```python
from build123d import *

# Parameters (mm, degrees)
BOSS_EXTRUDE1_DEPTH = 3.302
SKETCH3_R           = 5.08
CUT_EXTRUDE1_DEPTH  = 1.651
BOSS_EXTRUDE2_DEPTH = 4.445
SKETCH5_R           = 1.4605
BOSS_EXTRUDE3_DEPTH = 12.7


with BuildPart() as part:
    # Sketch1 → Boss-Extrude1 (new body)
    with BuildSketch(Plane(origin=(0, 0, 0), x_dir=(1, 0, 0), z_dir=(0, 1, 0))):
        with BuildLine():
            ThreePointArc((42.545, -8.433720508), (42.325290161, -7.400350502), (41.704170418, -6.545753376))
            Line((41.704170418, -6.545753376), (11.519480965, 20.620467131))
            ThreePointArc((11.519480965, 20.620467131), (10.730300515, 21.103895846), (9.820310547, 21.2725))
            Line((9.820310547, 21.2725), (-9.820310547, 21.2725))
            ThreePointArc((-9.820310547, 21.2725), (-10.730300515, 21.103895846), (-11.519480965, 20.620467131))
            Line((-11.519480965, 20.620467131), (-41.704170418, -6.545753376))
            ThreePointArc((-41.704170418, -6.545753376), (-42.325290161, -7.400350502), (-42.545, -8.433720508))
            Line((-42.545, -8.433720508), (-42.545, -16.8275))
            ThreePointArc((-42.545, -16.8275), (-41.243089642, -19.970589642), (-38.1, -21.2725))
            Line((-38.1, -21.2725), (-29.845, -21.2725))
            ThreePointArc((-29.845, -21.2725), (-26.701910358, -19.970589642), (-25.4, -16.8275))
            Line((-25.4, -16.8275), (-25.4, -16.3195))
            ThreePointArc((-25.4, -16.3195), (-23.912102448, -12.727397552), (-20.32, -11.2395))
            Line((-20.32, -11.2395), (-8.505751918, -11.2395))
            ThreePointArc((-8.505751918, -11.2395), (-7.87713399, -11.499882072), (-7.616751918, -12.1285))
            Line((-7.616751918, -12.1285), (-7.616751918, -15.9385))
            ThreePointArc((-7.616751918, -15.9385), (-7.505159602, -16.207907684), (-7.235751918, -16.3195))
            Line((-7.235751918, -16.3195), (6.099248082, -16.3195))
            ThreePointArc((6.099248082, -16.3195), (6.368655765, -16.207907684), (6.480248082, -15.9385))
            Line((6.480248082, -15.9385), (6.480248082, -12.1285))
            ThreePointArc((6.480248082, -12.1285), (6.740630153, -11.499882072), (7.369248082, -11.2395))
            Line((7.369248082, -11.2395), (20.32, -11.2395))
            ThreePointArc((20.32, -11.2395), (23.912102448, -12.727397552), (25.4, -16.3195))
            Line((25.4, -16.3195), (25.4, -16.8275))
            ThreePointArc((25.4, -16.8275), (26.701910358, -19.970589642), (29.845, -21.2725))
            Line((29.845, -21.2725), (38.1, -21.2725))
            ThreePointArc((38.1, -21.2725), (41.243089642, -19.970589642), (42.545, -16.8275))
            Line((42.545, -16.8275), (42.545, -8.433720508))
        make_face()
        with BuildLine():
            ThreePointArc((-38.735, -9.8425), (-38.288630735, -8.764869265), (-37.211, -8.3185))
            Line((-37.211, -8.3185), (-30.607, -8.3185))
            ThreePointArc((-30.607, -8.3185), (-29.529369265, -8.764869265), (-29.083, -9.8425))
            Line((-29.083, -9.8425), (-29.083, -16.1925))
            ThreePointArc((-29.083, -16.1925), (-29.529369265, -17.270130735), (-30.607, -17.7165))
            Line((-30.607, -17.7165), (-37.211, -17.7165))
            ThreePointArc((-37.211, -17.7165), (-38.288630735, -17.270130735), (-38.735, -16.1925))
            Line((-38.735, -16.1925), (-38.735, -9.8425))
        make_face(mode=Mode.SUBTRACT)
        with BuildLine():
            Line((30.734, -8.3185), (37.338, -8.3185))
            ThreePointArc((37.338, -8.3185), (38.415630735, -8.764869265), (38.862, -9.8425))
            Line((38.862, -9.8425), (38.862, -16.1925))
            ThreePointArc((38.862, -16.1925), (38.415630735, -17.270130735), (37.338, -17.7165))
            Line((37.338, -17.7165), (30.734, -17.7165))
            ThreePointArc((30.734, -17.7165), (29.656369265, -17.270130735), (29.21, -16.1925))
            Line((29.21, -16.1925), (29.21, -9.8425))
            ThreePointArc((29.21, -9.8425), (29.656369265, -8.764869265), (30.734, -8.3185))
        make_face(mode=Mode.SUBTRACT)
    extrude(amount=BOSS_EXTRUDE1_DEPTH)

    # Sketch3 → Cut-Extrude1 (cut)
    with BuildSketch(Plane(origin=(0, 3.302, 0), x_dir=(1, 0, 0), z_dir=(0, 1, 0))):
        with Locations(Location((-9.9695, 8.8265, 0), (0, 0, 270))):
            Circle(SKETCH3_R)
        with Locations(Location((9.9695, 8.8265, 0), (0, 0, 270))):
            Circle(SKETCH3_R)
    extrude(amount=-CUT_EXTRUDE1_DEPTH, mode=Mode.SUBTRACT)

    # Sketch4 → Boss-Extrude2 (add)
    with BuildSketch(Plane.XZ):
        with BuildLine():
            ThreePointArc((-20.1295, 8.4455), (0, 9.9695), (20.1295, 8.4455))
            Line((20.1295, 8.4455), (20.1295, -11.72845))
            Line((20.1295, -11.72845), (10.795, -20.1295))
            Line((10.795, -20.1295), (-10.795, -20.1295))
            Line((-10.795, -20.1295), (-20.1295, -11.72845))
            Line((-20.1295, -11.72845), (-20.1295, 8.4455))
        make_face()
    extrude(amount=BOSS_EXTRUDE2_DEPTH)

    # Sketch5 → Boss-Extrude3 (add)
    with BuildSketch(Plane(origin=(0, 3.302, 0), x_dir=(1, 0, 0), z_dir=(0, 1, 0))):
        with Locations(Location((-27.813, 0.3175, 0), (0, 0, 270))):
            Circle(SKETCH5_R)
    extrude(amount=BOSS_EXTRUDE3_DEPTH)


solid = part.part
```
The listing builds one solid part. Answer for the finished solid, in the listing's coordinates (mm). A direction names the side the tool comes from. Round coordinates to 2 decimals unless told otherwise and drop trailing zeros. Order: outer loops, then holes, each group sorted by start corner. A loop starts at its lowest first (then second) coordinate and runs counter-clockwise, first axis right, second up. Notation, with made-up numbers: (80, -33.75) -> (106, -33.75) arc R22 ccw to (106, -16.75) -> close; hole circle Ø5 at (40, 20.5). An arc over 180 degrees is marked (long way). Answer as CSV lines item,"result". Start each with the question number.
(1) The part is cut by section D-D (z = -17). Determine the outline of the cut face in (x, y) (3 decimals), then the cut area to 3 significant figures.
(2) Find the intervals of material crossed by probe 1 along Y at (x, z) = (15, -3) (3 decimals); probe 2 along Z at (x, y) = (0.5, -2.5); probe 3 along X at (y, z) = (-0.5, 1), in increasing order. Write a range as from..to.
(3) The part is cut by section B-B (x = -17). Determine the outline of the cut face in (y, z) (1 decimal).
(4) A tool of negligible diameter and unlimited length cuts with its end or side. For faces 1 (the face through (-15.397, -2.191, -15.988)), 2 (the face through (42.33, 1.63, 7.41)), 3 (the face through (29.668, 1.628, 17.282)), 4 (the face through (23.872, 1.628, 12.688)), from which of +Z, -Z, +X, -X, +Y, -Y can it reach the whole face along a straight path? Write none if from no direction.
(5) Flat-ended cylindrical pins translate along their axes: pin 1 Ø8 at (x, z) = (-9.5, -11) entering from +Y; pin 2 Ø1.7 at (x, y) = (35.5, 2) entering from -Z; pin 3 Ø1.3 at (y, z) = (-1.5, -2.5) entering from +X. Find the tip coordinate at first contact, or state that the pin passes through.
(6) The part is cut by section A-A (z = -6.5). Determine the outline of the cut face in (x, y) (1 decimal), then the cut area to 3 significant figures.
(7) For a pull along Z with two mould halves and no side action, classify faces 5 (the face through (-20.13, -2, -2)), 6 (the face through (15.006, 2.488, -9.488)), 7 (the face through (34, 2, 17.716)), 8 (the face through (0, -2, -20.13)) as +Z half, -Z half, draft (parallel to the pull), parting line (faces both ways), or undercut.
(8) The part is cut by section C-C (y = 6.75). Determine the outline of the cut face in (x, z), then the cut area to 3 significant figures.
Evaluation:
1,outline,"(-15.542, 0) -> (-14.272, 0) -> (-14.272, -4.445) -> (14.272, -4.445) -> (14.272, 0) -> (15.542, 0) -> (15.542, 3.302) -> (-15.542, 3.302) -> close"
1,area,"230 mm²"
2,probe 1,"-4.445..3.302"
2,probe 2,"-20.13..9.97"
2,probe 3,"-20.13..20.13"
3,outline,"(-4.4, -14.5) -> (0, -14.5) -> (0, -15.7) -> (3.3, -15.7) -> (3.3, 11.2) -> (0, 11.2) -> (0, 8.9) -> (-4.4, 8.9) -> close"
4,face 1,"-Z, -X, -Y"
4,face 2,"-Z, +X, +Y, -Y"
4,face 3,"+Y, -Y"
4,face 4,"+Z, +Y, -Y"
5,pin 1,"y = 3.3"
5,pin 2,"z = 0.2"
5,pin 3,"x = 20.13"
6,outline,"(-27.2, 0) -> (-20.1, 0) -> (-20.1, -4.4) -> (20.1, -4.4) -> (20.1, 0) -> (27.2, 0) -> (27.2, 3.3) -> (14.5, 3.3) -> (14.5, 1.7) -> (5.5, 1.7) -> (5.5, 3.3) -> (-5.5, 3.3) -> (-5.5, 1.7) -> (-14.5, 1.7) -> (-14.5, 3.3) -> (-27.2, 3.3) -> close"
6,area,"329 mm²"
7,face 5,"draft"
7,face 6,"undercut"
7,face 7,"undercut"
7,face 8,"-Z half"
8,outline,"circle Ø2.92 at (-27.81, -0.32)"
8,area,"6.70 mm²"
